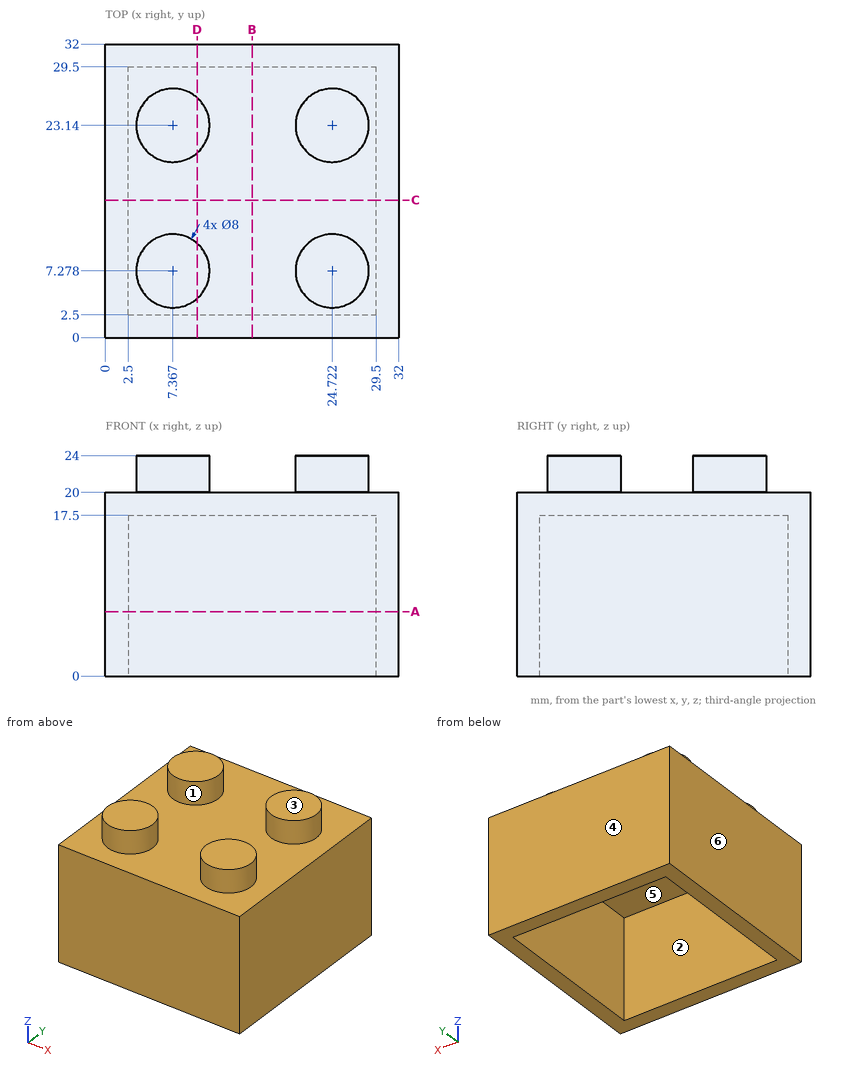
Job drawing, mm, ordinate dimensions from the low corner. One solid piece. A direction names the side the tool comes from. Give positions to 0.01 mm unless a question says otherwise; leave off trailing zeros. Write each loop counter-clockwise with the first axis right and the second up, starting at its lowest first coordinate (ties: lowest second). Pieces come first, ordered by that corner, then holes. Notation, with made-up numbers: M 75,83 L 86,83 A19 ccw 86,94 Z; hole C -30,71.25 d3. An arc over 180 degrees is marked long. One line per item, written item: value. Start each with the question number.
Q1. Saw through at B-B, the plane x = 16. Write the cut outline in (y, z).
Q2. Drop a flat-ended pin along its axis: pin 1 Ø1 at (x, y) = (18.5, 6) entering from -Z. Give the stop position or say it passes through.
Q3. 3-axis set-ups, long thin cutter, end or side, ignore diameter. For the marked faces 1, 2 and 3: which of +Z, -Z, +X, -X, +Y, -Y reach the whole face in a straight line?
Q4. Probe probe 1 along Y at (x, z) = (22, 6.5); probe 2 along Z at (x, y) = (7.5, 16). List the from-to ranges inside material, lowest first. Write a range as [from, to].
Q5. Saw through at D-D, the plane x = 10. Write the cut outline in (y, z), plus the area to 3 significant figures.
Q6. Two-plate mould, pull along X, no slides. Class the marked faces 4, 5 and 6: +X half, -X half, draft (parallel to the pull), parting line (faces both ways), or undercut.
Q7. Saw through at A-A, the plane z = 7. Write the cut outline in (x, y), plus the area to 3 significant figures.
Output values:
1. outline: M 0,0 L 2.5,0 L 2.5,17.5 L 29.5,17.5 L 29.5,0 L 32,0 L 32,20 L 0,20 Z
2. pin 1: stops at z = 17.5
3. face 1: +Z
3. face 2: -Z
3. face 3: +Z, +X, -X, +Y, -Y
4. probe 1: y = [0, 2.5], [29.5, 32]
4. probe 2: z = [17.5, 20]
5. outline: M 0,0 L 2.5,0 L 2.5,17.5 L 29.5,17.5 L 29.5,0 L 32,0 L 32,20 L 26.15,20 L 26.15,24 L 20.13,24 L 20.13,20 L 10.29,20 L 10.29,24 L 4.27,24 L 4.27,20 L 0,20 Z
5. area: 216 mm²
6. face 4: draft
6. face 5: undercut
6. face 6: -X half
7. outline: M 0,0 L 32,0 L 32,32 L 0,32 Z; hole M 2.5,2.5 L 29.5,2.5 L 29.5,29.5 L 2.5,29.5 Z
7. area: 295 mm²
